Input: part model. Units: mm. Frame: model coordinates. Face numbers are marked on the shaded views. A direction names the side the tool comes from. Round coordinates to 2 decimals unless told otherwise and drop trailing zeros. Loops run counter-clockwise (first coordinate to the right, second up) from the corner with the lowest first, then second, coordinate; pieces in that order, holes last. Notation, with made-up numbers: (3, 47.25) -> (23, 47.25) arc R30 ccw to (23, 73.25) -> close; hole circle Ø9 at (82, 18). An arc over 180 degrees is marked (long way). Answer in a Markdown table with one row per item. Add a question column.
Q1. Section A-A, the plane y = -36.83. Output: boundary loops of the cut face in (x, z) (3 decimals), and give its area (3 significant figures).
Q2. Ray query, L1, parallel to X at y = 19.05, z = 11.5 (3 decimals); L2, parallel to Y at x = 0, z = 2.9; L3, parallel to Z at x = 30, y = 5.5. Return the intervals inside material, ascending. Write a range as from..to.
Q3. Reachability of the marked faces 1, 2, 3 and 4 from +Z, -Z, +X, -X, +Y, -Y: full face, straight path, thin tool, end or side. Return the list, or none.
Q4. Section D-D, the plane y = 19.05. Output: boundary loops of the cut face in (x, z) (3 decimals).
Q5. Section B-B, the plane y = 0. Output: boundary loops of the cut face in (x, z) (3 decimals).
Q6. Pin query (flat end, axial travel): pin 1 (4 mm diameter, centred on y = 15, z = 17.5, fed in from -X) (3 decimals); pin 2 (5.5 mm diameter, centred on x = 0.5, y = -4, fed in from +Z); pin 3 (5 mm diameter, centred on x = 4.5, z = 10, fed in from -Y). Return the tip coordinate at first contact, or that it passes through.
Q7. Mould query, pull axis Z, two halves, no side actions, for the marked faces 5, 6, 7 and 8. Classes: pulls with the +Z half, pulls with the -Z half, needs draft (parallel to the pull), parting line crosses it, or undercut.
```python
from build123d import *
from build123d.topology import SkipClean

# Parameters (mm, degrees)
SKETCH1_R           = 57.15
BOSS_EXTRUDE1_DEPTH = 6.35
SKETCH1_5_R         = 62.23
SKETCH1_5_R_2       = 57.15
BOSS_EXTRUDE2_DEPTH = 4.445
SKETCH1_6_R         = 62.23
SKETCH1_6_R_2       = 57.15
CUT_EXTRUDE1_DEPTH  = 1.905
SKETCH1_12_R        = 12.7
SKETCH1_12_R_2      = 7.62
BOSS_EXTRUDE5_DEPTH = 69.85
SKETCH1_13_R        = 12.7
CUT_EXTRUDE3_DEPTH  = 3.81
SKETCH1_17_W        = 69.85
SKETCH1_17_H        = 76.2
SKETCH1_17_R        = 3.175
SKETCH1_17_R_2      = 12.7
SKETCH1_17_R_3      = 8.89
BOSS_EXTRUDE8_DEPTH = 19.05
SKETCH1_18_R        = 8.89
BOSS_EXTRUDE9_DEPTH = 22.86
SKETCH1_22_W        = 69.85
SKETCH1_22_H        = 76.2
SKETCH1_22_R        = 3.175
SKETCH1_22_R_2      = 12.7
SKETCH1_22_R_3      = 8.89
CUT_EXTRUDE6_DEPTH  = 2.54
FILLET1_R           = 2.54


with BuildPart() as part:
    # Sketch1 → Boss-Extrude1 (new body)
    with BuildSketch(Plane.XY):
        Circle(SKETCH1_R)
    extrude(amount=-BOSS_EXTRUDE1_DEPTH)

    # Sketch1_5 → Boss-Extrude2 (add)
    # profile 1 of 3: a face of its own
    with SkipClean():  # the faces are left unmerged after this step: merging them gives an invalid solid
        with BuildSketch(Plane.XY):
            Circle(SKETCH1_5_R)
            Circle(SKETCH1_5_R_2, mode=Mode.SUBTRACT)
        # profile 2 of 3: a face of its own
        with BuildSketch(Plane.XY):
            with BuildLine():
                Line((-34.925, -45.236786745), (-34.925, -50.8))
                Line((-34.925, -50.8), (-26.181720723, -50.8))
                ThreePointArc((-26.181720723, -50.8), (-30.679719112, -48.216981813), (-34.925, -45.236786745))
            make_face()
        # profile 3 of 3: a face of its own
        with BuildSketch(Plane.XY):
            with BuildLine():
                ThreePointArc((34.925, -45.236786745), (30.679719112, -48.216981813), (26.181720723, -50.8))
                Line((26.181720723, -50.8), (34.925, -50.8))
                Line((34.925, -50.8), (34.925, -45.236786745))
            make_face()
        extrude(amount=-BOSS_EXTRUDE2_DEPTH)

    # Sketch1_6 → Cut-Extrude1 (cut)
    # profile 1 of 3: a face of its own
    with SkipClean():  # the faces are left unmerged after this step: merging them gives an invalid solid
        with BuildSketch(Plane.XY):
            Circle(SKETCH1_6_R)
            Circle(SKETCH1_6_R_2, mode=Mode.SUBTRACT)
        # profile 2 of 3: a face of its own
        with BuildSketch(Plane.XY):
            with BuildLine():
                Line((-34.925, -45.236786745), (-34.925, -50.8))
                Line((-34.925, -50.8), (-26.181720723, -50.8))
                ThreePointArc((-26.181720723, -50.8), (-30.679719112, -48.216981813), (-34.925, -45.236786745))
            make_face()
        # profile 3 of 3: a face of its own
        with BuildSketch(Plane.XY):
            with BuildLine():
                ThreePointArc((34.925, -45.236786745), (30.679719112, -48.216981813), (26.181720723, -50.8))
                Line((26.181720723, -50.8), (34.925, -50.8))
                Line((34.925, -50.8), (34.925, -45.236786745))
            make_face()
        extrude(amount=-CUT_EXTRUDE1_DEPTH, mode=Mode.SUBTRACT)

    # Sketch1_12 → Boss-Extrude5 (add)
    # profile 1 of 2: a face of its own
    with SkipClean():  # the faces are left unmerged after this step: merging them gives an invalid solid
        with BuildSketch(Plane.XY):
            with Locations((0, -36.83)):
                Circle(SKETCH1_12_R)
            with Locations((0, -36.83)):
                Circle(SKETCH1_12_R_2, mode=Mode.SUBTRACT)
        # profile 2 of 2: a face of its own
        with BuildSketch(Plane.XY):
            with Locations((0, -36.83)):
                Circle(SKETCH1_12_R_2)
        extrude(amount=BOSS_EXTRUDE5_DEPTH)

    # Sketch1_13 → Cut-Extrude3 (cut)
    with SkipClean():  # the faces are left unmerged after this step: merging them gives an invalid solid
        with BuildSketch(Plane.XY):
            with Locations((0, -36.83)):
                Circle(SKETCH1_13_R)
        extrude(amount=CUT_EXTRUDE3_DEPTH, mode=Mode.SUBTRACT)


with BuildPart() as cut_extrude3_piece_1:
    # of the separate pieces the step leaves, piece 1, a body of its own (cut_extrude3_pieces)
    add(part.part.solids().sort_by_distance((57.15, 0, -4.445))[0])



with BuildPart() as cut_extrude3_piece_2:
    # of the separate pieces the step leaves, piece 2, a body of its own (cut_extrude3_pieces)
    add(part.part.solids().sort_by_distance((12.7, -36.83, 3.81))[0])


with BuildPart() as cut_extrude3_piece_1_1:
    with SkipClean():  # the faces are left unmerged after this step: merging them gives an invalid solid
        add(cut_extrude3_piece_1.part)

        add(cut_extrude3_piece_2.part)  # Boss-Extrude8 merges Cut-Extrude3 piece 2
        # Sketch1_17 → Boss-Extrude8 (add)
        with BuildSketch(Plane.XY):
            with Locations((0, -12.7)):
                Rectangle(SKETCH1_17_W, SKETCH1_17_H)
            with Locations(Location((-29.845, 19.05, 0), (0, 0, 180))):
                Circle(SKETCH1_17_R, mode=Mode.SUBTRACT)
            with Locations(Location((29.845, 19.05, 0), (0, 0, 180))):
                Circle(SKETCH1_17_R, mode=Mode.SUBTRACT)
            with Locations(Location((-29.845, -44.45, 0), (0, 0, 180))):
                Circle(SKETCH1_17_R, mode=Mode.SUBTRACT)
            with Locations(Location((29.845, -44.45, 0), (0, 0, 180))):
                Circle(SKETCH1_17_R, mode=Mode.SUBTRACT)
            with Locations((0, -36.83)):
                Circle(SKETCH1_17_R_2, mode=Mode.SUBTRACT)
            with Locations(Location((0, 0, 0), (0, 0, 180))):
                Circle(SKETCH1_17_R_3, mode=Mode.SUBTRACT)
        extrude(amount=BOSS_EXTRUDE8_DEPTH)

    # Sketch1_18 → Boss-Extrude9 (add)
    with SkipClean():  # the faces are left unmerged after this step: merging them gives an invalid solid
        with BuildSketch(Plane.XY):
            with Locations(Location((0, 0, 0), (0, 0, 180))):
                Circle(SKETCH1_18_R)
        extrude(amount=BOSS_EXTRUDE9_DEPTH)

    # Sketch1_22 → Cut-Extrude6 (cut)
    with SkipClean():  # the faces are left unmerged after this step: merging them gives an invalid solid
        with BuildSketch(Plane.XY):
            with Locations((0, -12.7)):
                Rectangle(SKETCH1_22_W, SKETCH1_22_H)
            with Locations(Location((29.845, 19.05, 0), (0, 0, 180))):
                Circle(SKETCH1_22_R, mode=Mode.SUBTRACT)
            with Locations(Location((-29.845, -44.45, 0), (0, 0, 180))):
                Circle(SKETCH1_22_R, mode=Mode.SUBTRACT)
            with Locations(Location((0, -36.83, 0), (0, 0, 180))):
                Circle(SKETCH1_22_R_2, mode=Mode.SUBTRACT)
            Circle(SKETCH1_22_R_3, mode=Mode.SUBTRACT)
            with Locations(Location((29.845, -44.45, 0), (0, 0, 180))):
                Circle(SKETCH1_22_R, mode=Mode.SUBTRACT)
            with Locations(Location((-29.845, 19.05, 0), (0, 0, 180))):
                Circle(SKETCH1_22_R, mode=Mode.SUBTRACT)
        extrude(amount=CUT_EXTRUDE6_DEPTH, mode=Mode.SUBTRACT)

    # Fillet1
    fillet1_edges = [cut_extrude3_piece_1_1.edges().sort_by_distance(p)[0] for p in [
        (-34.925, 25.4, 10.795),
        (-34.925, -50.8, 10.795),
        (34.925, -50.8, 10.795),
        (34.925, 25.4, 10.795),
    ]]
    fillet(fillet1_edges, radius=FILLET1_R)


solid = cut_extrude3_piece_1_1.part
```
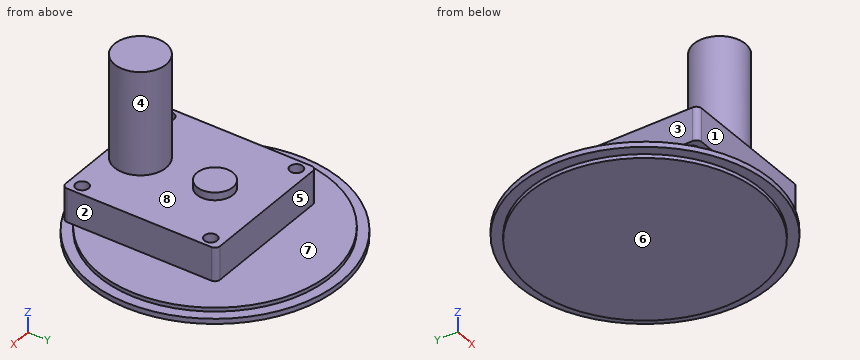
Answer block:
| question | item | result |
|---|---|---|
| 1 | outline | (-50.161, -4.445) -> (-43.7, -4.445) -> (-43.7, -6.35) -> (43.7, -6.35) -> (43.7, -4.445) -> (50.161, -4.445) -> (50.161, -1.905) -> (43.7, -1.905) -> (43.7, 0) -> (-43.7, 0) -> (-43.7, -1.905) -> (-50.161, -1.905) -> close; (-34.925, 2.54) -> (-12.7, 2.54) -> (-12.7, 3.81) -> (12.7, 3.81) -> (12.7, 2.54) -> (34.925, 2.54) -> (34.925, 19.05) -> (12.7, 19.05) -> (12.7, 69.85) -> (-12.7, 69.85) -> (-12.7, 19.05) -> (-34.925, 19.05) -> close |
| 1 | area | 3,000 mm^2 |
| 2 | L1 | -34.925..-33.02, -26.67..26.67, 33.02..34.925 |
| 2 | L2 | -50.8..-49.53, -24.13..25.4 |
| 2 | L3 | -6.35..0, 2.54..19.05 |
| 3 | face 1 | +Z, +X, -X, -Y |
| 3 | face 2 | +Z, +X, +Y, -Y |
| 3 | face 3 | +Z, -X, +Y, -Y |
| 3 | face 4 | +Z |
| 4 | outline | (-59.242, -4.445) -> (-53.882, -4.445) -> (-53.882, -6.35) -> (53.882, -6.35) -> (53.882, -4.445) -> (59.242, -4.445) -> (59.242, -1.905) -> (53.882, -1.905) -> (53.882, 0) -> (-53.882, 0) -> (-53.882, -1.905) -> (-59.242, -1.905) -> close; (-34.925, 2.54) -> (-33.02, 2.54) -> (-33.02, 19.05) -> (-34.925, 19.05) -> close; (-26.67, 2.54) -> (26.67, 2.54) -> (26.67, 19.05) -> (-26.67, 19.05) -> close; (33.02, 2.54) -> (34.925, 2.54) -> (34.925, 19.05) -> (33.02, 19.05) -> close |
| 5 | outline | (-62.23, -4.445) -> (-57.15, -4.445) -> (-57.15, -6.35) -> (57.15, -6.35) -> (57.15, -4.445) -> (62.23, -4.445) -> (62.23, -1.905) -> (57.15, -1.905) -> (57.15, 0) -> (8.89, 0) -> (8.89, 2.54) -> (34.925, 2.54) -> (34.925, 19.05) -> (8.89, 19.05) -> (8.89, 22.86) -> (-8.89, 22.86) -> (-8.89, 19.05) -> (-34.925, 19.05) -> (-34.925, 2.54) -> (-8.89, 2.54) -> (-8.89, 0) -> (-57.15, 0) -> (-57.15, -1.905) -> (-62.23, -1.905) -> close |
| 6 | pin 1 | x = -34.925 |
| 6 | pin 2 | z = 22.86 |
| 6 | pin 3 | y = -50.8 |
| 7 | face 5 | needs draft |
| 7 | face 6 | pulls with the -Z half |
| 7 | face 7 | undercut |
| 7 | face 8 | pulls with the +Z half |
